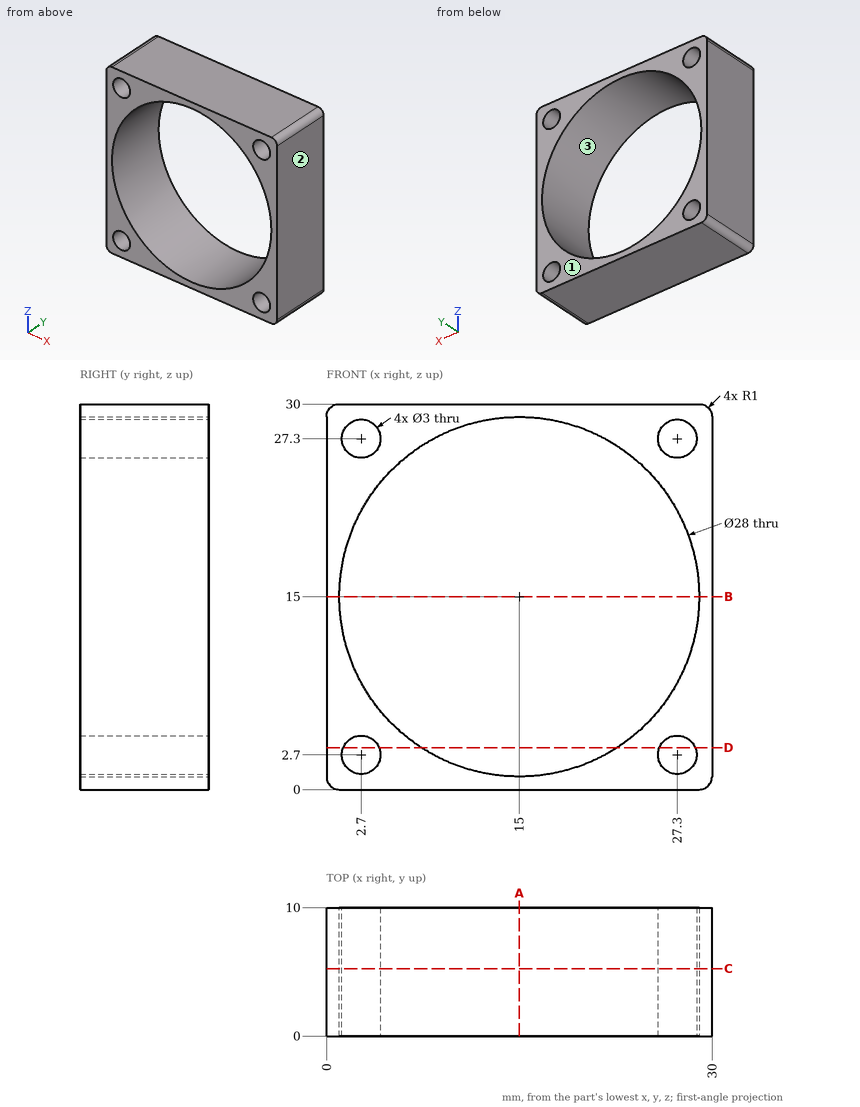
Geometry check sheet. Reference: drawing and pictorial views, mm from the part's lowest x, y, z. Round coordinates to 2 decimals unless told otherwise and drop trailing zeros. Loops run counter-clockwise (first coordinate to the right, second up) from the corner with the lowest first, then second, coordinate; pieces in that order, holes last. Notation, with made-up numbers: M 62,32 L 72,32 A17 ccw 72,63 Z; hole C 52.25,87 d3. An arc over 180 degrees is marked long. One line per item, written item: value.
(1) Thickness scan on line 1 (X direction, y = 8, z = 2.7); line 2 (X direction, y = 3, z = 15). Record the ranges inside material, lowest first.
Computed values:
line 1: x = 0 to 1.2, 4.2 to 8.31, 21.69 to 25.8, 28.8 to 30
line 2: x = 0 to 1, 29 to 30
(2) Depth check by flat-ended pin: pin 1 Ø2.5 at (x, z) = (27.3, 2.7) entering from +Y. Enter the tip coordinate at first touch or a pass-through.
Computed values:
pin 1: passes through
(3) Sectioned sample at C-C, the plane y = 5.25. Record the cut outline in (x, z).
Computed values:
outline: M 0,1 A1 ccw 1,0 L 29,0 A1 ccw 30,1 L 30,29 A1 ccw 29,30 L 1,30 A1 ccw 0,29 Z; hole C 15,15 d28; hole C 2.7,2.7 d3; hole C 2.7,27.3 d3; hole C 27.3,2.7 d3; hole C 27.3,27.3 d3
(4) Sectioned sample at B-B, the plane z = 15. Record the cut outline in (x, y), then the cut area to 3 significant figures.
Computed values:
outline: M 0,0 L 1,0 L 1,10 L 0,10 Z; M 29,0 L 30,0 L 30,10 L 29,10 Z
area: 20.0 mm^2
(5) Sectioned sample at D-D, the plane z = 3.25. Record the cut outline in (x, y), then the cut area to 3 significant figures.
Computed values:
outline: M 0,0 L 1.3,0 L 1.3,10 L 0,10 Z; M 4.1,0 L 7.39,0 L 7.39,10 L 4.1,10 Z; M 22.61,0 L 25.9,0 L 25.9,10 L 22.61,10 Z; M 28.7,0 L 30,0 L 30,10 L 28.7,10 Z
area: 91.9 mm^2
(6) Release check for a two-part mould opening along X. For the marked faces 1, 2 and 3 record: +X half, -X half, draft (parallel to the pull), parting line (faces both ways), or undercut.
Computed values:
face 1: draft
face 2: +X half
face 3: undercut
(7) Sectioned sample at A-A, the plane x = 15. Record the cut outline in (y, z).
Computed values:
outline: M 0,0 L 10,0 L 10,1 L 0,1 Z; M 0,29 L 10,29 L 10,30 L 0,30 Z
